The listing builds one solid part. Answer for the finished solid, in the listing's coordinates (mm). A direction names the side the tool comes from. Give positions to 0.01 mm unless a question says otherwise; leave off trailing zeros. Write each loop counter-clockwise with the first axis right and the second up, starting at its lowest first coordinate (ties: lowest second). Pieces come first, ordered by that corner, then holes. Notation, with made-up numbers: (77, -17.75) -> (96, -17.75) arc R21 cw to (96, 4.25) -> close; hole circle Ø7 at (85, -16.75). An arc over 180 degrees is marked (long way). One line per question, with ' | ' between items.
from build123d import *

# Parameters (mm, degrees)
F0_W     = 36.5
F0_H     = 45
F1_DEPTH = 7.13
F2_W     = 7
F2_H     = 40.08
F3_DEPTH = 7.13
F4_W     = 12.66
F4_H     = 36.17
F5_DEPTH = 7.13
F6_W     = 12.66
F6_H     = 3.91
F7_DEPTH = 3.53
F8_W     = 12.66
F8_H     = 4.8
F9_DEPTH = 3.5
F10_R    = 3


with BuildPart() as f1:
    # F0 (on Top) → F1 (new body)
    with BuildSketch(Plane.XY):
        with Locations((2.660514, 5.255292)):
            Rectangle(F0_W, F0_H)
    extrude(amount=F1_DEPTH)

    # F2 (on face) → F3 (cut)
    with BuildSketch(Plane.XY.offset(7.13)):
        with Locations((-12.089486, 7.715292)):
            Rectangle(F2_W, F2_H)
        with Locations((17.410514, 7.715292)):
            Rectangle(F2_W, F2_H)
    extrude(amount=-F3_DEPTH, mode=Mode.SUBTRACT)

    # F4 (on face) → F5 (cut)
    with BuildSketch(Plane.XY.offset(7.13)):
        with Locations((2.660514, 0.840292)):
            Rectangle(F4_W, F4_H)
    extrude(amount=-F5_DEPTH, mode=Mode.SUBTRACT)

    # F6 (on face) → F7 (cut)
    with BuildSketch(Plane.XY.offset(7.13)):
        with Locations((2.660514, 20.880292)):
            Rectangle(F6_W, F6_H)
    extrude(amount=-F7_DEPTH, mode=Mode.SUBTRACT)

    # F8 (on face) → F9 (join)
    with BuildSketch(Plane(origin=(0, 0, 0), x_dir=(1, 0, 0), z_dir=(0, 0, -1))):
        with Locations((2.660514, 6.474708)):
            Rectangle(F8_W, F8_H)
    extrude(amount=-F9_DEPTH)

    # F10
    f10_edges = [f1.edges().sort_by_distance(p)[0] for p in [
        (13.910514, -12.324708, 3.565),
        (-8.589486, -12.324708, 3.565),
    ]]
    fillet(f10_edges, radius=F10_R)


solid = f1.part
Item 1: Flat-ended cylindrical pins translate along their axes: pin 1 (5.5 mm diameter, centred on x = 5, y = -7, fed in from +Z); pin 2 (2 mm diameter, centred on y = 7, z = 5.5, fed in from -X); pin 3 (3 mm diameter, centred on x = 18.5, z = 3, fed in from +Y). Find the tip coordinate at first contact, or state that the pin passes through.
Answers below:
pin 1: z = 3.5 | pin 2: x = -8.59 | pin 3: y = -12.32
Item 2: Find section C-C (z = 1.5). Write down the section's boundary in (x, y).
Answers below:
outline: (-15.59, -17.24) -> (-3.67, -17.24) -> (-3.67, -8.87) -> (8.99, -8.87) -> (8.99, -17.24) -> (20.91, -17.24) -> (20.91, -12.32) -> (16.91, -12.32) arc R3 cw to (13.91, -9.32) -> (13.91, 27.76) -> (-8.59, 27.76) -> (-8.59, -9.32) arc R3 cw to (-11.59, -12.32) -> (-15.59, -12.32) -> close; hole (-3.67, -4.07) -> (8.99, -4.07) -> (8.99, 18.93) -> (-3.67, 18.93) -> close
Item 3: Find section D-D (y = -6). Write down the section's boundary in (x, z).
Answers below:
outline: (-8.59, 0) -> (13.91, 0) -> (13.91, 7.13) -> (8.99, 7.13) -> (8.99, 3.5) -> (-3.67, 3.5) -> (-3.67, 7.13) -> (-8.59, 7.13) -> close
Item 4: A tool of negligible diameter and unlimited length cuts with its end or side. For faces 1 (the face through (3, 21, 3.6)), 2 (the face through (3, -4.075, 2)), 3 (the face through (-3.669, 3, 4)), 4 (the face through (19, -12.325, 4)), 5 (the face through (-14, -12.325, 4)), from which of +Z, -Z, +X, -X, +Y, -Y can it reach the whole face along a straight path? Write none if from no direction.
Answers below:
face 1: +Z, -Y | face 2: +Z, -Z | face 3: +Z | face 4: +Z, -Z, +X, +Y | face 5: +Z, -Z, -X, +Y
Item 5: Find section A-A (y = 17). Write down the section's boundary in (x, z), then the cut area to 3 significant figures.
Answers below:
outline: (-8.59, 0) -> (-3.67, 0) -> (-3.67, 7.13) -> (-8.59, 7.13) -> close; (8.99, 0) -> (13.91, 0) -> (13.91, 7.13) -> (8.99, 7.13) -> close | area: 70.2 mm²
Item 6: Find section B-B (x = 3). Write down the section's boundary in (y, z).
Answers below:
outline: (-8.87, 0) -> (-4.07, 0) -> (-4.07, 3.5) -> (-8.87, 3.5) -> close; (18.93, 0) -> (27.76, 0) -> (27.76, 7.13) -> (22.84, 7.13) -> (22.84, 3.6) -> (18.93, 3.6) -> close
Item 7: Determine the mould class of faces 6 (the face through (3, 22.835, 5)), 7 (the face through (14.766, -11.423, 3.515)), 8 (the face through (-8.589, 9, 4)), 9 (the face through (15, -17.245, 4)) for opening direction X: pulls with the +X half, pulls with the -X half, needs draft (parallel to the pull), parting line crosses it, or undercut.
Answers below:
face 6: undercut | face 7: pulls with the +X half | face 8: pulls with the -X half | face 9: needs draft
Item 8: Consider line 1 (X direction, y = 19, z = 5); line 2 (X direction, y = -14, z = 3.75); line 3 (Y direction, x = 1, z = 1.5). Determine where each line is inside the solid, lowest interval first. Write a range as [from, to].
Answers below:
line 1: [-8.59, -3.67], [8.99, 13.91] | line 2: [-15.59, -3.67], [8.99, 20.91] | line 3: [-8.87, -4.07], [18.93, 27.76]
